Part model, mm, in its own coordinate system. Face numbers are marked on the shaded views. A direction names the side the tool comes from. Round coordinates to 2 decimals unless told otherwise and drop trailing zeros. Loops run counter-clockwise (first coordinate to the right, second up) from the corner with the lowest first, then second, coordinate; pieces in that order, holes last. Notation, with made-up numbers: M 30.25,89 L 62.25,89 A35 cw 62.25,123 Z; hole C 47,28 d10. An arc over 180 degrees is marked long. Put each result on its own line as item: value. Start each with the question number.
1) Slice it at A-A on y = 15.75. Give the cut face in (x, z).
2) Slice it at C-C on y = 21.5. Give the cut face in (x, z).
3) Which spindle directions (+Z, -Z, +X, -X, +Y, -Y) get a long thin tool onto all of the face, cutting with end or side? Do the marked faces 1 and 2. Say none if no direction does.
4) Probe line 1 along X through (y, z) = (4, -1.1); line 2 along Y through (x, z) = (12, -1.4); line 3 along Y through (x, z) = (15, -1.7). List the from-to ranges inside material, lowest first.
5) Slice it at D-D on x = 11.75. Give the cut face in (y, z), then the cut area to 3 significant figures.
6) Slice it at B-B on z = -0.65. Give the cut face in (x, y), then the cut area to 3 significant figures.
7) Drop a flat-ended pin along its axis: pin 1 Ø0.6 at (x, z) = (10.5, -1) entering from -Y. Give the stop position or say it passes through.
8) Pull direction X, two halves, no side cores. Call the marked faces 3, 4 and 5: +X half, -X half, draft (parallel to the pull), parting line (faces both ways), or undercut.
```python
from build123d import *

# Parameters (mm, degrees)
SKETCH1_W           = 2
SKETCH1_H           = 2
BOSS_EXTRUDE1_DEPTH = 24
SKETCH2_W           = 2
SKETCH2_H           = 2
BOSS_EXTRUDE2_DEPTH = 16
SKETCH3_W           = 2
SKETCH3_H           = 2
BOSS_EXTRUDE3_DEPTH = 22
FILLET1_R           = 2
FILLET2_R           = 2


with BuildPart() as part:
    # Sketch1 → Boss-Extrude1 (new body)
    with BuildSketch(Plane(origin=(0, 0, 0), x_dir=(1, 0, 0), z_dir=(0, 1, 0))):
        with Locations((1, 1)):
            Rectangle(SKETCH1_W, SKETCH1_H)
    extrude(amount=BOSS_EXTRUDE1_DEPTH)

    # Sketch2 → Boss-Extrude2 (add)
    with BuildSketch(Plane(origin=(2, 0, 0), x_dir=(0, 0, -1), z_dir=(1, 0, 0))):
        with Locations((1, 23)):
            Rectangle(SKETCH2_W, SKETCH2_H)
    extrude(amount=BOSS_EXTRUDE2_DEPTH)

    # Sketch3 → Boss-Extrude3 (add)
    with BuildSketch(Plane(origin=(0, 22, 0), x_dir=(-1, 0, 0), z_dir=(0, -1, 0))):
        with Locations((-17, 1)):
            Rectangle(SKETCH3_W, SKETCH3_H)
    extrude(amount=BOSS_EXTRUDE3_DEPTH)

    # Fillet1
    fillet1_edges = [part.edges().sort_by_distance(p)[0] for p in [
        (2, 22, -1),
        (16, 22, -1),
    ]]
    fillet(fillet1_edges, radius=FILLET1_R)

    # Fillet2
    fillet2_edges = [part.edges().sort_by_distance(p)[0] for p in [
        (18, 24, -1),
        (0, 24, -1),
    ]]
    fillet(fillet2_edges, radius=FILLET2_R)


solid = part.part
```
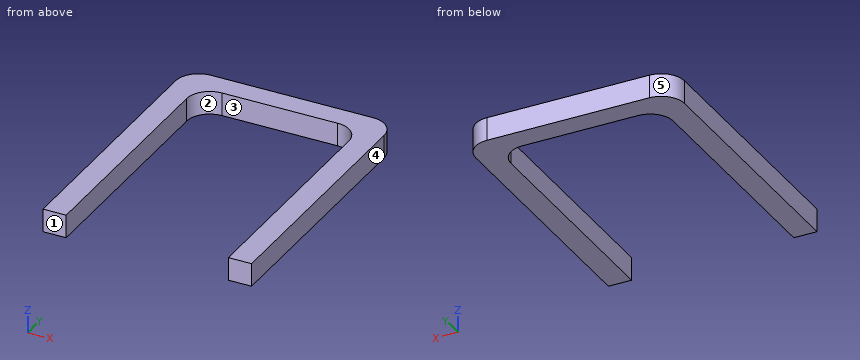
Recorded:
1. outline: M 0,-2 L 2,-2 L 2,0 L 0,0 Z; M 16,-2 L 18,-2 L 18,0 L 16,0 Z
2. outline: M 0,-2 L 2.68,-2 L 2.68,0 L 0,0 Z; M 15.32,-2 L 18,-2 L 18,0 L 15.32,0 Z
3. face 1: +Z, -Z, +X, -X, -Y
3. face 2: +Z, -Z, -Y
4. line 1: x = 0 to 2, 16 to 18
4. line 2: y = 22 to 24
4. line 3: y = 21.73 to 24
5. outline: M 22,-2 L 24,-2 L 24,0 L 22,0 Z
5. area: 4.00 mm2
6. outline: M 0,0 L 2,0 L 2,20 A2 cw 4,22 L 14,22 A2 cw 16,20 L 16,0 L 18,0 L 18,22 A2 ccw 16,24 L 2,24 A2 ccw 0,22 Z
6. area: 124 mm2
7. pin 1: stops at y = 22
8. face 3: undercut
8. face 4: +X half
8. face 5: -X half
